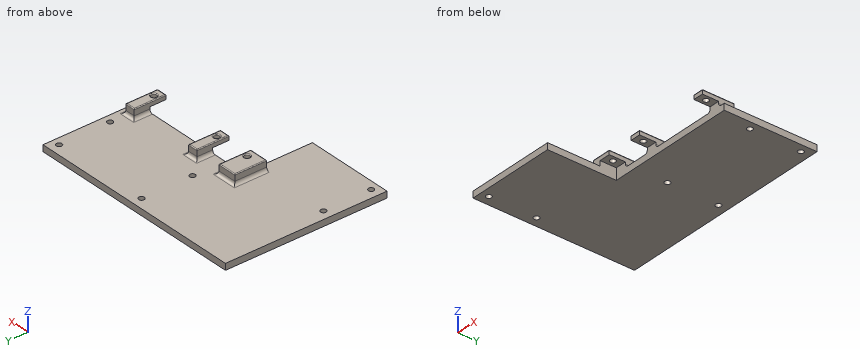
from build123d import *

# Parameters (mm, degrees)
SKETCH_1_W          = 138.25
SKETCH_1_H          = 101.5
EXTRUDE_1_DEPTH     = 4
SKETCH_2_W          = 81.75
SKETCH_2_H          = 43.2
CUT_EXTRUDE_1_DEPTH = 5
SKETCH_3_R          = 1.75
CUT_EXTRUDE_2_DEPTH = 5
SKETCH_4_W          = 6.4
SKETCH_4_H          = 20
SKETCH_4_R          = 1.75
SKETCH_4_W_2        = 12
EXTRUDE_6_DEPTH     = 6
FILLET_3_R          = 2
SKETCH_5_W          = 3.2
SKETCH_5_H          = 10.2
CUT_EXTRUDE_3_DEPTH = 81.75
FILLET_4_R          = 0.5


with BuildPart() as part:
    # ｽｹｯﾁ1 → ﾎﾞｽ - 押し出し1 (new body)
    with BuildSketch(Plane.XY):
        Rectangle(SKETCH_1_W, SKETCH_1_H)
    extrude(amount=EXTRUDE_1_DEPTH)

    # ｽｹｯﾁ2 → ｶｯﾄ - 押し出し1 (cut, through all)
    with BuildSketch(Plane.XY.offset(4)):
        with Locations((28.25, -29.15)):
            Rectangle(SKETCH_2_W, SKETCH_2_H)
    extrude(amount=-CUT_EXTRUDE_1_DEPTH, mode=Mode.SUBTRACT)

    # ｽｹｯﾁ3 → ｶｯﾄ - 押し出し2 (cut, through all)
    with BuildSketch(Plane.XY.offset(4)):
        with Locations((-63.125, -45.75)):
            Circle(SKETCH_3_R)
        with Locations((-63.125, -15.75)):
            Circle(SKETCH_3_R)
        with Locations((64.125, 44.75)):
            Circle(SKETCH_3_R)
        with Locations((64.125, 12.75)):
            Circle(SKETCH_3_R)
        with Locations((1.625, 44.75)):
            Circle(SKETCH_3_R)
        with Locations((1.625, 12.75)):
            Circle(SKETCH_3_R)
    extrude(amount=-CUT_EXTRUDE_2_DEPTH, mode=Mode.SUBTRACT)

    # ｽｹｯﾁ4 → ﾎﾞｽ - 押し出し6 (add)
    with BuildSketch(Plane.XY.offset(4)):
        with Locations((61.675, -7.75)):
            Rectangle(SKETCH_4_W, SKETCH_4_H)
        with Locations((61.675, -12.75)):
            Circle(SKETCH_4_R, mode=Mode.SUBTRACT)
        with Locations((14.075, -7.75)):
            Rectangle(SKETCH_4_W, SKETCH_4_H)
        with Locations((14.075, -12.75)):
            Circle(SKETCH_4_R, mode=Mode.SUBTRACT)
        with Locations((-11.725, -7.75)):
            Rectangle(SKETCH_4_W_2, SKETCH_4_H)
        with Locations((-8.925, -12.75)):
            Circle(SKETCH_4_R, mode=Mode.SUBTRACT)
    extrude(amount=EXTRUDE_6_DEPTH)

    # ﾌｨﾚｯﾄ3
    fillet_3_edges = [part.edges().sort_by_distance(p)[0] for p in [
        (64.875, -2.65, 4),
        (61.675, 2.25, 4),
        (58.475, -2.65, 4),
        (17.275, -2.65, 4),
        (14.075, 2.25, 4),
        (10.875, -2.65, 4),
        (-5.725, -2.65, 4),
        (-11.725, 2.25, 4),
        (-17.725, -7.75, 4),
    ]]
    fillet(fillet_3_edges, radius=FILLET_3_R)

    # ｽｹｯﾁ5 → ｶｯﾄ - 押し出し3 (cut)
    with BuildSketch(Plane(origin=(69.125, 0, 0), x_dir=(0, 0, -1), z_dir=(1, 0, 0))):
        with Locations((-5.6, -12.65)):
            Rectangle(SKETCH_5_W, SKETCH_5_H)
    extrude(amount=-CUT_EXTRUDE_3_DEPTH, mode=Mode.SUBTRACT)

    # ﾌｨﾚｯﾄ4
    fillet_4_edges = [part.edges().sort_by_distance(p)[0] for p in [
        (64.875, -7.75, 10),
        (61.675, 2.25, 10),
        (58.475, -7.75, 10),
        (61.675, -17.75, 10),
        (59.925, -12.75, 10),
        (17.275, -7.75, 10),
        (14.075, 2.25, 10),
        (10.875, -7.75, 10),
        (14.075, -17.75, 10),
        (12.325, -12.75, 10),
        (-5.725, -7.75, 10),
        (-11.725, 2.25, 10),
        (-17.725, -7.75, 10),
        (-11.725, -17.75, 10),
        (-10.675, -12.75, 10),
    ]]
    fillet(fillet_4_edges, radius=FILLET_4_R)


solid = part.part
Work out the finished part from the listing and answer in its coordinate system (mm). Give positions to 0.01 mm unless a question says otherwise; leave off trailing zeros. Order: outer loops, then holes, each group sorted by start corner. A loop starts at its lowest first (then second) coordinate and runs counter-clockwise, first axis right, second up. Notation, with made-up numbers: (75, 72) -> (94, 72) arc R29 cw to (94, 99) -> close; hole circle Ø8 at (-39, 53). An arc over 180 degrees is marked (long way). Answer as a JSON object with one key per item and string values. Group by question number.
1. Section A-A on y = -45.75 is taken. Determine the outline of the cut face in (x, z) (3 decimals), plus the area to 3 significant figures.
2. Section B-B on y = 44.75 is taken. Determine the outline of the cut face in (x, z) (3 decimals), plus the area to 3 significant figures.
3. Section C-C on z = 1.5 is taken. Determine the outline of the cut face in (x, y) (3 decimals).
4. Section D-D on x = 28 is taken. Determine the outline of the cut face in (y, z), plus the area to 3 significant figures.
5. Consider line 1 along X through (y, z) = (-16.5, 8.5) (3 decimals); line 2 along X through (y, z) = (-12.75, 8.7) (3 decimals); line 3 along X through (y, z) = (-2, 5.5). Determine where each line is inside the solid, lowest interval first. Write a range as [from, to].
6. Flat-ended cylindrical pins translate along their axes: pin 1 Ø4 at (y, z) = (-10, 8.5) entering from -X (3 decimals); pin 2 Ø3 at (x, y) = (15.5, -14.5) entering from -Z; pin 3 Ø3 at (y, z) = (-6, 7.5) entering from +X (3 decimals). Find the tip coordinate at first contact, or state that the pin passes through.
Result sheet:
{
 "1": {"outline": "(-69.125, 0) -> (-64.875, 0) -> (-64.875, 4) -> (-69.125, 4) -> close; (-61.375, 0) -> (-12.625, 0) -> (-12.625, 4) -> (-61.375, 4) -> close", "area": "212 mm^2"},
 "2": {"outline": "(-69.125, 0) -> (-0.125, 0) -> (-0.125, 4) -> (-69.125, 4) -> close; (3.375, 0) -> (62.375, 0) -> (62.375, 4) -> (3.375, 4) -> close; (65.875, 0) -> (69.125, 0) -> (69.125, 4) -> (65.875, 4) -> close", "area": "525 mm^2"},
 "3": {"outline": "(-69.125, -50.75) -> (-12.625, -50.75) -> (-12.625, -7.55) -> (69.125, -7.55) -> (69.125, 50.75) -> (-69.125, 50.75) -> close; hole circle Ø3.5 at (-63.125, -45.75); hole circle Ø3.5 at (-63.125, -15.75); hole circle Ø3.5 at (1.625, 12.75); hole circle Ø3.5 at (1.625, 44.75); hole circle Ø3.5 at (64.125, 12.75); hole circle Ø3.5 at (64.125, 44.75)"},
 "4": {"outline": "(-7.55, 0) -> (50.75, 0) -> (50.75, 4) -> (-7.55, 4) -> close", "area": "233 mm^2"},
 "5": {"line 1": "x = [-17.725, -5.725], [10.875, 17.275], [58.475, 64.875]", "line 2": "x = [-17.725, -10.675], [-7.175, -5.725], [10.875, 12.325], [15.825, 17.275], [58.475, 59.925], [63.425, 64.875]", "line 3": "x = [-17.79, -5.66], [10.81, 17.34], [58.41, 64.94]"},
 "6": {"pin 1": "stops at x = -17.725", "pin 2": "stops at z = 7.2", "pin 3": "stops at x = 64.875"}
}
